from build123d import *

# Parameters (mm, degrees)
BOSS_EXTRUDE1_DEPTH = 1.5
SKETCH2_R           = 2.95
BOSS_EXTRUDE2_DEPTH = 8
SKETCH3_R           = 2.95
BOSS_EXTRUDE3_DEPTH = 92


with BuildPart() as part:
    # Sketch1 → Boss-Extrude1 (new body)
    with BuildSketch(Plane.XY):
        with BuildLine():
            Line((0, 5), (140, 5))
            ThreePointArc((140, 5), (145, 0), (140, -5))
            Line((140, -5), (0, -5))
            ThreePointArc((0, -5), (-5, 0), (0, 5))
        make_face()
    extrude(amount=BOSS_EXTRUDE1_DEPTH)

    # Sketch2 → Boss-Extrude2 (add)
    with BuildSketch(Plane.XY.offset(1.5)):
        Circle(SKETCH2_R)
        with Locations((140, 0)):
            Circle(SKETCH2_R)
    extrude(amount=BOSS_EXTRUDE2_DEPTH)

    # Sketch3 → Boss-Extrude3 (add)
    with BuildSketch(Plane.XY.offset(9.5)):
        Circle(SKETCH3_R)
    extrude(amount=BOSS_EXTRUDE3_DEPTH)


solid = part.part
The listing builds one solid part. Answer for the finished solid, in the listing's coordinates (mm). A direction names the side the tool comes from. Give positions to 0.01 mm unless a question says otherwise; leave off trailing zeros. Loops run counter-clockwise (first coordinate to the right, second up) from the corner with the lowest first, then second, coordinate; pieces in that order, holes last. Notation, with made-up numbers: (20, 74) - (70, 74) arc R28 ccw to (70, 96) - close; hole circle Ø10 at (40, 43.25). An arc over 180 degrees is marked (long way). Answer as a JSON object with one key per item and string values.
1. For a pull along X with two mould halves and no side action, classify faces 1 (the cylindrical face through (142.814, 0.886, 5.444)), 2 (the cylindrical face through (145, 0, 1)), 3 (the flat face through (140, 0, 9.5)) as pulls with the +X half, pulls with the -X half, needs draft (parallel to the pull), parting line crosses it, or undercut.
Determined:
{"face 1": "undercut", "face 2": "pulls with the +X half", "face 3": "needs draft"}
2. A cutting plane is placed at B-B (z = 26.5). Write down the section's boundary in (x, y).
Determined:
{"outline": "circle Ø5.9 at (0, 0)"}
3. Find the intervals of material crossed by L1, parallel to X at y = -0.25, z = 27; L2, parallel to Z at x = 92.5, y = 1.75; L3, parallel to X at y = -1, z = 80.5, in increasing order. Write a range as [from, to].
Determined:
{"L1": "[-2.94, 2.94]", "L2": "[0, 1.5]", "L3": "[-2.78, 2.78]"}
4. Flat-ended cylindrical pins translate along their axes: pin 1 Ø2 at (y, z) = (3.5, 32) entering from -X; pin 2 Ø3 at (y, z) = (3.5, 40) entering from +X; pin 3 Ø4 at (x, y) = (88, -1.5) entering from +Z. Find the tip coordinate at first contact, or state that the pin passes through.
Determined:
{"pin 1": "x = -1.57", "pin 2": "x = 2.17", "pin 3": "z = 1.5"}
5. For faces 4 (the cylindrical face through (-2.947, 0.13, 50.8)), 5 (the flat face through (71, 0, 0)), determine the directions among +Z, -Z, +X, -X, +Y, -Y from which every point of the face is accessible in a straight line to the end or side of a thin tool.
Determined:
{"face 4": "+Z", "face 5": "-Z, +X, -X, +Y, -Y"}
6. A cutting plane is placed at A-A (y = 0). Write down the section's boundary in (x, z), then the cut area to 3 significant figures.
Determined:
{"outline": "(-5, 0) - (145, 0) - (145, 1.5) - (142.95, 1.5) - (142.95, 9.5) - (137.05, 9.5) - (137.05, 1.5) - (2.95, 1.5) - (2.95, 101.5) - (-2.95, 101.5) - (-2.95, 1.5) - (-5, 1.5) - close", "area": "862 mm²"}
7. A cutting plane is placed at C-C (x = 87.5). Write down the section's boundary in (y, z), then the cut area to 3 significant figures.
Determined:
{"outline": "(-5, 0) - (5, 0) - (5, 1.5) - (-5, 1.5) - close", "area": "15.0 mm²"}
